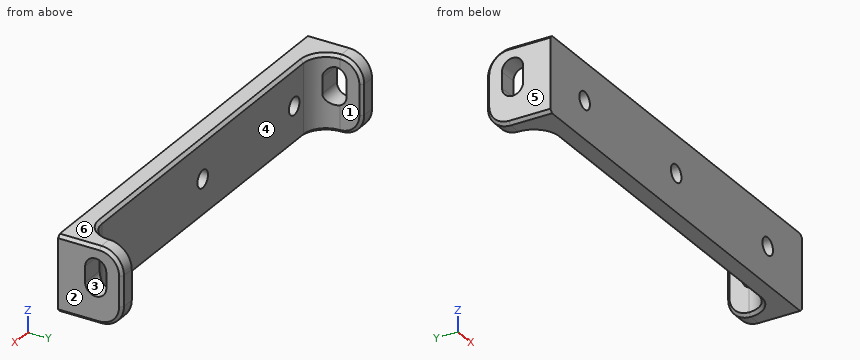
```python
from build123d import *

# Parameters (mm, degrees)
BOSS_EXTRUDE1_DEPTH = 25.4
FILLET1_R           = 7.62
SKETCH2_R           = 2.921
CUT_EXTRUDE1_DEPTH  = 143.805838816
CHAMFER1_SIZE       = 1.016
CUT_EXTRUDE2_DEPTH  = 144.622345406


with BuildPart() as part:
    # Sketch1 → Boss-Extrude1 (new body)
    with BuildSketch(Plane.XY):
        Polygon((0, 0), (0, 21.59), (6.35, 21.59), (6.35, 6.35), (133.35, 6.35), (133.35, 21.59), (139.7, 21.59), (139.7, 0), align=None)
    extrude(amount=BOSS_EXTRUDE1_DEPTH)

    # Fillet1
    fillet1_edges = [part.edges().sort_by_distance(p)[0] for p in [
        (136.525, 21.59, 0),
        (136.525, 21.59, 25.4),
        (3.175, 21.59, 0),
        (3.175, 21.59, 25.4),
        (133.35, 6.35, 12.7),
        (6.35, 6.35, 12.7),
    ]]
    fillet(fillet1_edges, radius=FILLET1_R - 0.0001)  # a hair under: the kernel refuses the full size

    # Sketch2 → Cut-Extrude1 (cut, through all)
    with BuildSketch(Plane(origin=(0, 6.35, 0), x_dir=(1, 0, 0), z_dir=(0, 1, 0))):
        with Locations(Location((69.85, -12.7, 0), (0, 0, 270))):
            Circle(SKETCH2_R)
        with Locations(Location((120.65, -12.7, 0), (0, 0, 270))):
            Circle(SKETCH2_R)
        with Locations(Location((19.05, -12.7, 0), (0, 0, 270))):
            Circle(SKETCH2_R)
    extrude(amount=-CUT_EXTRUDE1_DEPTH, mode=Mode.SUBTRACT)

    # Chamfer1
    chamfer1_edges = [part.edges().sort_by_distance(p)[0] for p in [
        (139.7, 6.98505, 0),
        (133.35, 21.59, 12.7),
        (139.7, 21.59, 12.7),
        (133.35, 19.358182962, 23.168182962),
        (133.35, 19.358182962, 2.231817038),
        (0, 6.98505, 0),
        (69.85, 6.35, 0),
        (139.7, 19.358182962, 23.168182962),
        (139.7, 19.358182962, 2.231817038),
        (69.85, 6.35, 25.4),
        (0, 6.98505, 25.4),
        (0, 21.59, 12.7),
        (6.35, 21.59, 12.7),
        (0, 19.358182962, 23.168182962),
        (0, 19.358182962, 2.231817038),
        (6.35, 19.358182962, 23.168182962),
        (6.35, 19.358182962, 2.231817038),
        (131.118182962, 8.581817038, 0),
        (131.118182962, 8.581817038, 25.4),
        (8.581817038, 8.581817038, 0),
        (8.581817038, 8.581817038, 25.4),
        (139.7, 6.98505, 25.4),
    ]]
    chamfer(chamfer1_edges, length=CHAMFER1_SIZE)

    # Sketch3 → Cut-Extrude2 (cut, through all)
    with BuildSketch(Plane(origin=(139.7, 0, 0), x_dir=(0, 0, -1), z_dir=(1, 0, 0))):
        with BuildLine():
            Line((-17.78, 16.256), (-12.446, 16.256))
            ThreePointArc((-12.446, 16.256), (-8.89, 12.7), (-12.446, 9.144))
            Line((-12.446, 9.144), (-17.78, 9.144))
            ThreePointArc((-17.78, 9.144), (-21.336, 12.7), (-17.78, 16.256))
        make_face()
    extrude(amount=-CUT_EXTRUDE2_DEPTH, mode=Mode.SUBTRACT)


solid = part.part
```
The listing builds one solid part. Answer for the finished solid, in the listing's coordinates (mm). Face numbers are marked on the shaded views. A direction names the side the tool comes from. Round coordinates to 2 decimals unless told otherwise and drop trailing zeros. Loops run counter-clockwise (first coordinate to the right, second up) from the corner with the lowest first, then second, coordinate; pieces in that order, holes last. Notation, with made-up numbers: (-30, -1.5) - (5, -1.5) arc R13 cw to (5, 19.5) - close; hole circle Ø11 at (23.25, -37.5). An arc over 180 degrees is marked (long way). Use one line per item in the form item = value. Start each with the question number.
1. Consider line 1 (X direction, y = 4, z = 12.7); line 2 (X direction, y = 17.5, z = 6); line 3 (Y direction, x = 115, z = 24.25). Determine where each line is inside the solid, lowest interval first. Write a range as [from, to].
2. For a pull along X with two mould halves and no side action, classify the marked faces 4, 5 and 6 as pulls with the +X half, pulls with the -X half, needs draft (parallel to the pull), parting line crosses it, or undercut.
3. The part is cut by section A-A on x = 69.85. Determine the outline of the cut face in (y, z), then the cut area to 3 significant figures.
4. A tool of negligible diameter and unlimited length cuts with its end or side. For the marked faces 1, 2 and 3, from which of +Z, -Z, +X, -X, +Y, -Y can it reach the whole face along a straight path? Write none if from no direction.
5. The part is cut by section B-B on z = 14.25. Give the number of separate pieces and of enclosed holes in the cut face, then the cut area to 3 significant figures.
6. Given pin 1 Ø2 at (x, z) = (54.5, 12) entering from +Y, flat-ended and moving along its own axis, determine where the tip first touches the part or whether it passes through.
Geometry check:
q1.line_1 = [0, 16.13], [21.97, 66.93], [72.77, 117.73], [123.57, 139.7]
q1.line_2 = [0, 6.35], [133.35, 139.7]
q1.line_3 = [0, 6.35]
q2.face_4 = undercut
q2.face_5 = pulls with the -X half
q2.face_6 = needs draft
q3.outline = (0, 0) - (5.33, 0) - (6.35, 1.02) - (6.35, 9.78) - (0, 9.78) - close; (0, 15.62) - (6.35, 15.62) - (6.35, 24.38) - (5.33, 25.4) - (0, 25.4) - close
q3.area = 123 mm^2
q4.face_1 = +Z, -Z, +Y
q4.face_2 = +Z, -Z, +X, +Y, -Y
q4.face_3 = +X, -X
q5.separate_pieces = 6
q5.enclosed_holes = 0
q5.area = 914 mm^2
q6.pin_1 = 6.35
